Check sheet for the modelled part. Datum: model origin and axes. Units: mm. A direction names the side the tool comes from. Round coordinates to 2 decimals unless told otherwise and drop trailing zeros. Write each loop counter-clockwise with the first axis right and the second up, starting at its lowest first coordinate (ties: lowest second). Pieces come first, ordered by that corner, then holes. Notation, with made-up numbers: (82, 89.5) -> (130, 89.5) arc R23 cw to (130, 115.5) -> close; hole circle Ø8 at (55.25, 66.5). An arc over 180 degrees is marked (long way). Answer as a JSON object with one key per item and string values. Group by question number.
```python
from build123d import *

# Parameters (mm, degrees)
SKETCH_2_R          = 6
CUT_EXTRUDE_1_DEPTH = 27
CUT_EXTRUDE_2_DEPTH = 4
CHAMFER_3_SIZE      = 1
CHAMFER_4_SIZE      = 0.5


with BuildPart() as part:
    # 草图1 → 旋转1 (revolve)
    with BuildSketch(Plane.XY):
        Polygon((0, 0), (9, 0), (9, 15), (8, 15), (8, 16), (8, 16.5), (10, 16.5), (10, 16), (13, 16), (13, 17), (15, 17), (15, 26), (0, 26), align=None)
    revolve(axis=Axis((0, 26, 0), (0, -1, 0)))

    # 草图2 → 切除-拉伸1 (cut, through all)
    with BuildSketch(Plane.XZ):
        Circle(SKETCH_2_R)
    extrude(amount=-CUT_EXTRUDE_1_DEPTH, mode=Mode.SUBTRACT)

    # 草图3 → 切除-拉伸2 (cut)
    with BuildSketch(Plane(origin=(0, 26, 0), x_dir=(1, 0, 0), z_dir=(0, 1, 0))):
        with BuildLine():
            Line((11, 10.198039027), (11, -10.198039027))
            ThreePointArc((11, -10.198039027), (15, 0), (11, 10.198039027))
        make_face()
    extrude(amount=-CUT_EXTRUDE_2_DEPTH, mode=Mode.SUBTRACT)

    # 倒角3
    chamfer_3_edges = [part.edges().sort_by_distance(p)[0] for p in [
        (-9, 0, 0),
        (-15, 17, 0),
        (-6, 26, 0),
        (-15, 26, 0),
    ]]
    chamfer(chamfer_3_edges, length=CHAMFER_3_SIZE)

    # 倒角4
    chamfer_4_edges = [part.edges().sort_by_distance(p)[0] for p in [
        (-9, 15, 0),
        (-6, 0, 0),
    ]]
    chamfer(chamfer_4_edges, length=CHAMFER_4_SIZE)


solid = part.part
```
(1) Section check A-A on y = 19.25. Record the cut outline in (x, z).
(2) Go/stop test with flat-tipped pins: pin 1 Ø1 at (x, z) = (-8.5, 1) entering from -Y; pin 2 Ø1.5 at (x, z) = (10, -9.5) entering from -Y; pin 3 Ø1 at (x, z) = (0, 11.5) entering from -Y. Record where each tip stops, or that it passes through.
(3) Release check for a two-part mould opening along X. For faces 5 (the cylindrical face through (-2.17, 16.25, -9.76)), 6 (the flat face through (-7, 16, -8)), 7 (the cylindrical face through (-1.172, 7.844, 8.923)) record: pulls with the +X half, pulls with the -X half, needs draft (parallel to the pull), parting line crosses it, or undercut.
(4) Section check B-B on y = 12.25. Record the cut outline in (x, z), then the cut area to 3 significant figures.
(5) Access from +Z, -Z, +X, -X, +Y, -Y to the whole of each face (thin tool, end or side, straight path). Record for faces 1 (the conical face through (-14.165, 25.826, 0.491)), 2 (the flat face through (11, 24, 0)), 3 (the cylindrical face through (-1.73, 15.76, -7.81)), 4 (the cylindrical face through (-10.316, 16.507, -7.91)).
(6) Scan lines: line 1 along Z through (x, y) = (0, 16.35); line 2 along Z through (x, y) = (0, 15.75); line 3 along X through (y, z) = (23.25, 4.5). Record each from-to range of solid material in increasing order.
Data:
{
 "1": {"outline": "circle Ø30 at (0, 0); hole circle Ø12 at (0, 0)"},
 "2": {"pin 1": "stops at y = 0.06", "pin 2": "stops at y = 17", "pin 3": "stops at y = 16"},
 "3": {"face 5": "undercut", "face 6": "needs draft", "face 7": "parting line crosses it"},
 "4": {"outline": "circle Ø18 at (0, 0); hole circle Ø12 at (0, 0)", "area": "141 mm²"},
 "5": {"face 1": "+Y", "face 2": "+Z, -Z, +X, +Y", "face 3": "none", "face 4": "-Y"},
 "6": {"line 1": "z = -13 to -10, -8 to -6, 6 to 8, 10 to 13", "line 2": "z = -8 to -6, 6 to 8", "line 3": "x = -14.31 to -3.97, 3.97 to 11"}
}
